Drawing for the job (mm, zero at the part's lowest x, y, z). Round coordinates to 2 decimals unless told otherwise and drop trailing zeros. Write each loop counter-clockwise with the first axis right and the second up, starting at its lowest first coordinate (ties: lowest second). Pieces come first, ordered by that corner, then holes. Notation, with made-up numbers: (35.25, 84) - (61.25, 84) arc R34 cw to (61.25, 118) - close; hole circle Ø8 at (-39, -24). An arc over 180 degrees is marked (long way). Answer in a Markdown table with one row per item.
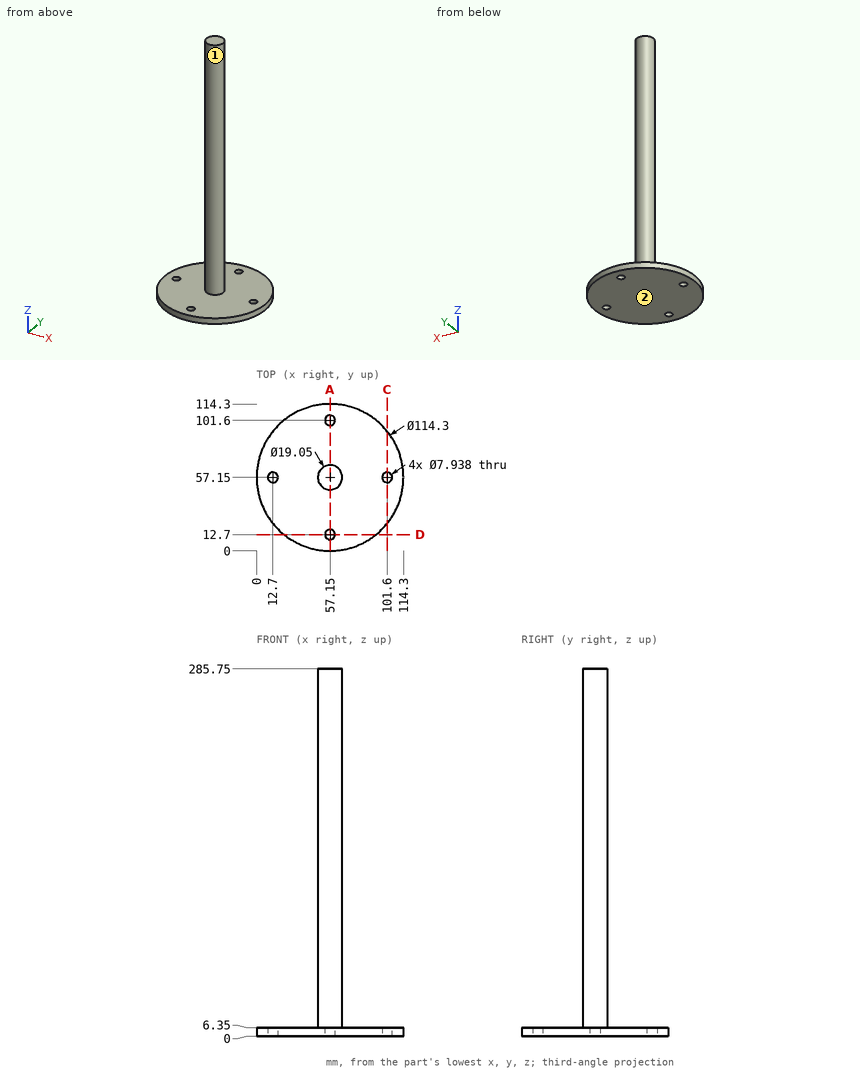
Q1. Saw through at C-C on x = 101.6. List the corners of the cut face in (y, z).
Computed:
| item | result |
|---|---|
| outline | (21.23, 0) - (53.18, 0) - (53.18, 6.35) - (21.23, 6.35) - close; (61.12, 0) - (93.07, 0) - (93.07, 6.35) - (61.12, 6.35) - close |
Q2. Drill centre lines: line 1 (Y direction, x = 57.15, z = 2.25); line 2 (X direction, y = 57, z = 5) (1 decimal); line 3 (Z direction, x = 68.5, y = 92). Where is each one in solid material? Low to high.
Computed:
| item | result |
|---|---|
| line 1 | y = 0 to 8.73, 16.67 to 97.63, 105.57 to 114.3 |
| line 2 | x = 0 to 8.7, 16.7 to 97.6, 105.6 to 114.3 |
| line 3 | z = 0 to 6.35 |
Q3. Pull direction Y, two halves, no side cores. Call the marked faces 1 and 2: released by +Y, released by -Y, zero draft, split by the parting line, or undercut.
Computed:
| item | result |
|---|---|
| face 1 | split by the parting line |
| face 2 | zero draft |
Q4. Flat gauge pins, fed straight in: pin 1 (5 mm diameter, centred on x = 101.6, y = 57.15, fed in from +Z); pin 2 (10.5 mm diameter, centred on x = 57.15, y = 12.7, fed in from -Z); pin 3 (10 mm diameter, centred on x = 20, y = 76, fed in from +Z). Where does each tip first touch, or does it go through?
Computed:
| item | result |
|---|---|
| pin 1 | passes through |
| pin 2 | stops at z = 0 |
| pin 3 | stops at z = 6.35 |
Q5. Saw through at A-A on x = 57.15. Count the separate pieces of the cut face and the enclosed holes in it, then the cut area to 3 significant figures.
Computed:
| item | result |
|---|---|
| separate pieces | 3 |
| enclosed holes | 0 |
| area | 5,950 mm2 |
